```python
from build123d import *

# Parameters (mm, degrees)
F0_R                 = 4.445
F1_DEPTH             = 5.08
F2_R                 = 4.445
F3_DEPTH             = 25.4
F4_R                 = 4.318
F5_DEPTH             = 25.4
F8_D                 = 6.35
F8_DEPTH             = 22.86
F8_CBORE_D           = 6.35
F8_CBORE_DEPTH       = 12.7
F8_TIP               = 1.9077324654
F8_ON_F7_D           = 6.35
F8_ON_F7_DEPTH       = 22.86
F8_ON_F7_CBORE_D     = 6.35
F8_ON_F7_CBORE_DEPTH = 12.7
F8_ON_F7_TIP         = 1.9077324654


with BuildPart() as f1:
    # F0 (on Front) → F1 (new body)
    with BuildSketch(Plane.XZ):
        with BuildLine():
            Line((16.9093859117, 17.425267489), (27.1303756598, 27.6462572371))
            ThreePointArc((27.1303756598, 27.6462572371), (33.2640046568, 38.2700142946), (22.6402475993, 32.1363852977))
            Line((22.6402475993, 32.1363852977), (12.4192578512, 21.9153955495))
            Line((12.4192578512, 21.9153955495), (12.4192578512, 36.5455265367))
            Line((12.4192578512, 36.5455265367), (12.4192578512, 55.5955265367))
            Line((12.4192578512, 55.5955265367), (-30.3997510844, 55.5955265367))
            Line((-30.3997510844, 55.5955265367), (-30.3997510844, 36.5455265367))
            Line((-30.3997510844, 36.5455265367), (-44.8762217871, 36.5455265367))
            ThreePointArc((-44.8762217871, 36.5455265367), (-56.7254831011, 33.3705265367), (-44.8762217871, 30.1955265367))
            Line((-44.8762217871, 30.1955265367), (-30.3997510844, 30.1955265367))
            Line((-30.3997510844, 30.1955265367), (-30.3997510844, 16.4088443772))
            Line((-30.3997510844, 16.4088443772), (-30.3997510844, 10.0526214838))
            Line((-30.3997510844, 10.0526214838), (-15.6116463411, 10.0526214838))
            Line((-15.6116463411, 10.0526214838), (-6.5234490096, 2.9726886888))
            Line((-6.5234490096, 2.9726886888), (-13.581341862, -4.0852041636))
            ThreePointArc((-13.581341862, -4.0852041636), (-19.714970859, -14.7089612211), (-9.0912138015, -8.5753322242))
            Line((-9.0912138015, -8.5753322242), (-2.033320949, -1.5174393717))
            Line((-2.033320949, -1.5174393717), (5.046611846, -10.6056367033))
            Line((5.046611846, -10.6056367033), (5.046611846, -25.3937414465))
            Line((5.046611846, -25.3937414465), (11.4028347394, -25.3937414465))
            Line((11.4028347394, -25.3937414465), (25.1895168989, -25.3937414465))
            Line((25.1895168989, -25.3937414465), (25.1895168989, -39.8702121492))
            ThreePointArc((25.1895168989, -39.8702121492), (28.3645168989, -51.7194734633), (31.5395168989, -39.8702121492))
            Line((31.5395168989, -39.8702121492), (31.5395168989, -25.3937414465))
            Line((31.5395168989, -25.3937414465), (50.5895168989, -25.3937414465))
            Line((50.5895168989, -25.3937414465), (50.5895168989, 17.425267489))
            Line((50.5895168989, 17.425267489), (31.5395168989, 17.425267489))
            Line((31.5395168989, 17.425267489), (16.9093859117, 17.425267489))
        make_face()
        with Locations((22.6495168989, -7.2694734633)):
            Circle(F0_R, mode=Mode.SUBTRACT)
        with Locations((-12.2754831011, 27.6555265367)):
            Circle(F0_R, mode=Mode.SUBTRACT)
    extrude(amount=F1_DEPTH)

    # F2 (on face) → F3 (join)
    with BuildSketch(Plane.XZ.offset(5.08)):
        with Locations((-12.2754831011, 27.6555265367)):
            Circle(F2_R)
        with Locations((22.6495168989, -7.2694734633)):
            Circle(F2_R)
    extrude(amount=-F3_DEPTH)

    # F4 (on face) → F5 (cut)
    with BuildSketch(Plane(origin=(0, 0, 0), x_dir=(-1, 0, 0), z_dir=(0, 1, 0))):
        with Locations((-28.7738765962, 33.7798862341)):
            Circle(F4_R)
        with Locations((15.2248427984, -10.2188331606)):
            Circle(F4_R)
        with Locations((50.3754831011, 33.3705265367)):
            Circle(F4_R)
        with Locations((-28.3645168989, -45.3694734633)):
            Circle(F4_R)
    extrude(amount=-F5_DEPTH, mode=Mode.SUBTRACT)

    # F8
    with Locations(Plane(origin=(0, 20.32, 0), x_dir=(-1, 0, 0), z_dir=(0, 1, 0))):
        with Locations((-22.6495168989, -7.2694734633)):
            CounterBoreHole(F8_D / 2, F8_CBORE_D / 2, F8_CBORE_DEPTH, depth=F8_DEPTH)
            with Locations((0, 0, -(F8_DEPTH + F8_TIP / 2))):  # 118° drill point
                Cone(0, F8_D / 2, F8_TIP, mode=Mode.SUBTRACT)

    # F8 on F7
    with Locations(Plane(origin=(0, 20.32, 0), x_dir=(-1, 0, 0), z_dir=(0, 1, 0))):
        with Locations((12.2754831011, 27.6555265367)):
            CounterBoreHole(F8_ON_F7_D / 2, F8_ON_F7_CBORE_D / 2, F8_ON_F7_CBORE_DEPTH, depth=F8_ON_F7_DEPTH)
            with Locations((0, 0, -(F8_ON_F7_DEPTH + F8_ON_F7_TIP / 2))):  # 118° drill point
                Cone(0, F8_ON_F7_D / 2, F8_ON_F7_TIP, mode=Mode.SUBTRACT)


solid = f1.part
```
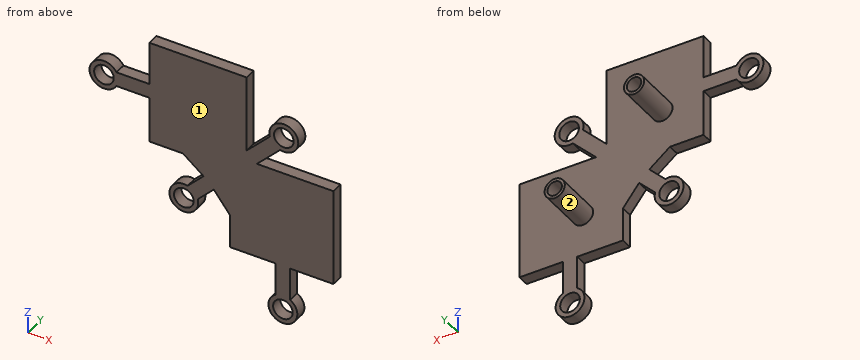
Check sheet for the modelled part. Datum: model origin and axes. Units: mm. Face numbers are marked on the shaded views. A direction names the side the tool comes from. Round coordinates to 2 decimals unless told otherwise and drop trailing zeros. Loops run counter-clockwise (first coordinate to the right, second up) from the corner with the lowest first, then second, coordinate; pieces in that order, holes last. Notation, with made-up numbers: M 36.25,80 L 78.25,80 A15 ccw 78.25,84 Z; hole C -2,-19 d4. An arc over 180 degrees is marked long. Answer as a JSON object with one key per item and string values.
1. Section check C-C (z = 14). Record the boundary of the cut face in (x, y), plus the area to 3 significant figures.
Reply:
{"outline": "M -30.4,-5.08 L 50.59,-5.08 L 50.59,0 L -30.4,0 Z", "area": "411 mm²"}
2. Scan lines: line 1 (X direction, y = -2.5, z = -38); line 2 (Y direction, x = -9.5, z = 16); line 3 (X direction, y = 9, z = -4.5). Record each from-to range of solid material in increasing order.
Reply:
{"line 1": "x = 25.19 to 31.54", "line 2": "y = -5.08 to 0", "line 3": "x = 19.17 to 21.1, 24.2 to 26.13"}
3. Section check D-D (x = -23). Record the boundary of the cut face in (y, z), plus the area to 3 significant figures.
Reply:
{"outline": "M -5.08,10.05 L 0,10.05 L 0,55.6 L -5.08,55.6 Z", "area": "231 mm²"}
4. Section check A-A (x = 29). Record the boundary of the cut face in (y, z), plus the area to 3 significant figures.
Reply:
{"outline": "M -5.08,-51.69 L 0,-51.69 L 0,-49.64 L -5.08,-49.64 Z; M -5.08,-41.1 L 0,-41.1 L 0,17.43 L -5.08,17.43 Z; M -5.08,27.43 L 0,27.43 L 0,29.47 L -5.08,29.47 Z; M -5.08,38.09 L 0,38.09 L 0,40.13 L -5.08,40.13 Z", "area": "328 mm²"}
5. Access from +Z, -Z, +X, -X, +Y, -Y to the whole of each face (thin tool, end or side, straight path). Record for the marked faces 1 and 2.
Reply:
{"face 1": "+Z, -Z, +X, -X, -Y", "face 2": "+Y"}
6. Gauge pin test, flat ends, axial feed: P1, Ø3, axis at x = -24.5, y = 2.5, coming from the +Z side; P2, Ø5.5, axis at x = 45, y = -2, coming from the -Z side; P3, Ø4, axis at x = 22.65, z = -7.27, coming from the +Y side; P4, Ø3, axis at y = 4, z = 32, coming from the +X side. Record the tip position at first contact, or that the pin passes through.
Reply:
{"P1": "passes through", "P2": "stops at z = -25.39", "P3": "stops at y = -3.25", "P4": "stops at x = -8.86"}
7. Section check B-B (y = 9.5). Record the boundary of the cut face in (x, z) (3 decimals).
Reply:
{"outline": "C -12.275,27.656 d8.89; C 22.65,-7.269 d8.89; hole C -12.275,27.656 d6.35; hole C 22.65,-7.269 d6.35"}
